Can you work these out from the model? Positions are in its coordinate system, mm. A direction names the side the tool comes from. Round coordinates to 2 decimals unless told otherwise and drop trailing zeros. Loops run counter-clockwise (first coordinate to the right, second up) from the corner with the lowest first, then second, coordinate; pieces in that order, holes last.
from build123d import *
from OCP.BRepFilletAPI import BRepFilletAPI_MakeChamfer

# Parameters (mm, degrees)
BOSS_EXTRUDE1_DEPTH             = 2
BOSS_EXTRUDE2_REACH             = 41.681
SKETCH2_W                       = 18.31765306
SKETCH2_H                       = 6
BOSS_EXTRUDE2_DIRECTION_2_DEPTH = 10
CUT_EXTRUDE1_DEPTH              = 8
CUT_EXTRUDE2_DEPTH              = 39.837136106
CUT_EXTRUDE2_DEPTH_BACK         = 39.837136106
SKETCH4_W                       = 8
SKETCH4_H                       = 2
CHAMFER1_SIZE                   = 2
CHAMFER2_SIZE                   = 10
CHAMFER2_SIZE2                  = 5.773502692
FILLET1_START                   = -2
FILLET1_DEPTH                   = 4
FILLET1_2_DEPTH                 = 4
BOSS_EXTRUDE3_START             = -6
SKETCH5_W                       = 10
SKETCH5_H                       = 1.6
BOSS_EXTRUDE3_DEPTH             = 10.5


with BuildPart() as part:
    # Sketch1 → Boss-Extrude1 (new, symmetric)
    with BuildSketch(Plane(origin=(0, 0, 0), x_dir=(1, 0, 0), z_dir=(0, 1, 0))):
        Polygon((-8, 0), (0, 0), (0, -1.2), (-9.15882653, -1.2), (-9.606841403, 11.62946737), (-13.196767517, 17.374550089), (-21.640774961, 32), (-20.255134315, 32), (-12.168010072, 17.992689924), (-8.41879396, 11.992689924), align=None)
    boss_extrude1 = extrude(amount=BOSS_EXTRUDE1_DEPTH, both=True)

    # Mirror1: Boss-Extrude1 across plane
    add(boss_extrude1.mirror(Plane(origin=(0, 2, 0), x_dir=(0, 0, 1), z_dir=(-1, 0, 0))))

    # Boss-Extrude2: up to this face of the body (flat: up to its plane)
    boss_extrude2_end = Plane(part.part.faces().sort_by_distance((0, 0, 0))[0])
    # Sketch2 → Boss-Extrude2 (add, up to the picked face)
    with BuildSketch(Plane.XY.offset(1.2), mode=Mode.PRIVATE) as boss_extrude2_sk1:
        with Locations((0, -1)):
            Rectangle(SKETCH2_W, SKETCH2_H)
    boss_extrude2_tool1 = split(extrude(boss_extrude2_sk1.sketch, amount=-BOSS_EXTRUDE2_REACH, mode=Mode.PRIVATE), bisect_by=boss_extrude2_end, keep=Keep.BOTH, mode=Mode.PRIVATE)
    add(boss_extrude2_tool1.solids().sort_by(Axis((0, -1, 1.2), (0, 0, -1)))[0])

    # Sketch2 → Boss-Extrude2 direction 2 (add)
    with BuildSketch(Plane.XY.offset(1.2)):
        with Locations((0, -1)):
            Rectangle(SKETCH2_W, SKETCH2_H)
    extrude(amount=BOSS_EXTRUDE2_DIRECTION_2_DEPTH)

    # Sketch3 → Cut-Extrude1 (cut)
    with BuildSketch(Plane.XY.offset(11.2)):
        with BuildLine():
            Line((-1.5, 1.826658805), (-1.5, 2))
            Line((-1.5, 2), (1.5, 2))
            Line((1.5, 2), (1.5, 1.826658805))
            ThreePointArc((1.5, 1.826658805), (3.2, -1), (1.5, -3.826658805))
            Line((1.5, -3.826658805), (1.5, -4))
            Line((1.5, -4), (-1.5, -4))
            Line((-1.5, -4), (-1.5, -3.826658805))
            ThreePointArc((-1.5, -3.826658805), (-3.2, -1), (-1.5, 1.826658805))
        make_face()
    extrude(amount=-CUT_EXTRUDE1_DEPTH, mode=Mode.SUBTRACT)

    # Sketch4 → Cut-Extrude2 (cut, two sides: drawn at the far end of the back side and taken through both)
    with BuildSketch(Plane(origin=(0, 0, 0), x_dir=(1, 0, 0), z_dir=(0, 1, 0)).offset(-CUT_EXTRUDE2_DEPTH_BACK)):
        with Locations((0, -4.2)):
            Rectangle(SKETCH4_W, SKETCH4_H)
    extrude(amount=CUT_EXTRUDE2_DEPTH + CUT_EXTRUDE2_DEPTH_BACK, mode=Mode.SUBTRACT)

    # Chamfer1
    chamfer1_edges = [part.edges().sort_by_distance(p)[0] for p in [
        (8.579413265, -2, 0),
        (-8.579413265, -2, 0),
    ]]
    chamfer(chamfer1_edges, length=CHAMFER1_SIZE - 0.0001)  # a hair under: the kernel refuses the full size

    # Chamfer2: one chamfer whose edges measure the first distance from different faces: ONE call of the kernel's chamfer builder (chamfer() names one face for all edges)
    chamfer2_edges_1 = [part.edges().sort_by_distance(p)[0] for p in [
        (9.15882653, -1, 11.2),
    ]]
    chamfer2_side_1 = [part.faces().sort_by_distance(p)[0] for p in [
        (9.15882653, -1.126288177, 5.77807488),
    ]]
    chamfer2_edges_2 = [part.edges().sort_by_distance(p)[0] for p in [
        (-9.15882653, -1, 11.2),
    ]]
    chamfer2_side_2 = [part.faces().sort_by_distance(p)[0] for p in [
        (-9.15882653, -1.126288177, 5.77807488),
    ]]
    chamfer2 = BRepFilletAPI_MakeChamfer(part.part.solid().wrapped)
    for e in chamfer2_edges_1:
        chamfer2.Add(CHAMFER2_SIZE, CHAMFER2_SIZE2, e.wrapped, chamfer2_side_1[0].wrapped)  # the first distance lies on this face
    for e in chamfer2_edges_2:
        chamfer2.Add(CHAMFER2_SIZE, CHAMFER2_SIZE2, e.wrapped, chamfer2_side_2[0].wrapped)  # the first distance lies on this face
    add(Compound.cast(chamfer2.Shape()), mode=Mode.REPLACE)

    # Fillet1: read off the stored shape, not the designer's step
    # Fillet1 outline → Fillet1 (cut)
    with BuildSketch(Plane(origin=(0, 0, 0), x_dir=(1, 0, 0), z_dir=(0, 1, 0)).offset(FILLET1_START)):
        with BuildLine():
            Line((13.196767517, 17.374550089), (13.327680504, 17.601298033))
            ThreePointArc((13.327680504, 17.601298033), (13.194808958, 17.37572691), (13.05802089, 17.15250907))
            Line((13.05802089, 17.15250907), (13.196767517, 17.374550089))
        make_face()
        with BuildLine():
            ThreePointArc((8.278524581, 7.975900449), (8.924815647, 11.837983569), (10.548665544, 15.401196962))
            Line((10.548665544, 15.401196962), (8.41879396, 11.992689924))
            Line((8.41879396, 11.992689924), (8.278524581, 7.975900449))
        make_face()
        with BuildLine():
            Line((-13.196767517, 17.374550089), (-13.05802089, 17.15250907))
            ThreePointArc((-13.05802089, 17.15250907), (-13.194808958, 17.37572691), (-13.327680504, 17.601298033))
            Line((-13.327680504, 17.601298033), (-13.196767517, 17.374550089))
        make_face()
        with BuildLine():
            Line((-8.41879396, 11.992689924), (-10.548665544, 15.401196962))
            ThreePointArc((-10.548665544, 15.401196962), (-8.924815647, 11.837983569), (-8.278524581, 7.975900449))
            Line((-8.278524581, 7.975900449), (-8.41879396, 11.992689924))
        make_face()
    extrude(amount=FILLET1_DEPTH, mode=Mode.SUBTRACT)

    # Fillet1 2 outline → Fillet1 2 (add)
    with BuildSketch(Plane(origin=(0, 0, 0), x_dir=(1, 0, 0), z_dir=(0, 1, 0)).offset(FILLET1_START)):
        with BuildLine():
            ThreePointArc((9.466572023, 7.612677895), (10.112863089, 11.474761015), (11.736712986, 15.037974408))
            Line((11.736712986, 15.037974408), (9.606841403, 11.62946737))
            Line((9.606841403, 11.62946737), (9.466572023, 7.612677895))
        make_face()
        with BuildLine():
            ThreePointArc((12.298923059, 18.219437869), (12.166051513, 17.993866745), (12.029263444, 17.770648906))
            Line((12.029263444, 17.770648906), (12.168010072, 17.992689924))
            Line((12.168010072, 17.992689924), (12.298923059, 18.219437869))
        make_face()
        with BuildLine():
            Line((-9.606841403, 11.62946737), (-11.736712986, 15.037974408))
            ThreePointArc((-11.736712986, 15.037974408), (-10.112863089, 11.474761015), (-9.466572023, 7.612677895))
            Line((-9.466572023, 7.612677895), (-9.606841403, 11.62946737))
        make_face()
        with BuildLine():
            ThreePointArc((-12.029263444, 17.770648906), (-12.166051513, 17.993866745), (-12.298923059, 18.219437869))
            Line((-12.298923059, 18.219437869), (-12.168010072, 17.992689924))
            Line((-12.168010072, 17.992689924), (-12.029263444, 17.770648906))
        make_face()
    extrude(amount=FILLET1_2_DEPTH)

    # Sketch5 → Boss-Extrude3 (add)
    with BuildSketch(Plane.XZ.offset(4).offset(BOSS_EXTRUDE3_START)):
        with Locations((0, 0.8)):
            Rectangle(SKETCH5_W, SKETCH5_H)
    extrude(amount=BOSS_EXTRUDE3_DEPTH)


solid = part.part
(1) If we section it at D-D, the plane z = -22: List the corners of the cut face in (x, y) for me, then the cut area to 3 significant figures.
Worked answers:
outline: (-15.87, -2) - (-14.48, -2) - (-14.48, 2) - (-15.87, 2) - close; (14.48, -2) - (15.87, -2) - (15.87, 2) - (14.48, 2) - close
area: 11.1 mm2
(2) If we mould it in two halves opening along Z, with no side actions, what happens to faces 1 (the flat face through (-3.6, -1, 5.2)), 2 (the flat face through (0, -4, 3)), 3 (the flat face through (17.426, 0.028, -24.7))? For each: released by +Z, released by -Z, zero draft, split by the parting line, or undercut.
Worked answers:
face 1: undercut
face 2: zero draft
face 3: released by +Z
(3) Will these pins go through, and if not, where does the flat tip stop? P1, Ø2, axis at y = -1, z = 4, coming from the -X side; P2, Ø3, axis at y = -7, z = -1, coming from the -X side; P3, Ø2, axis at y = -3.5, z = 0.5, coming from the -X side.
Worked answers:
P1: stops at x = -8.12
P2: stops at x = -5
P3: stops at x = -9.16
(4) If we section it at B-B, the plane z = 4: List the corners of the cut face in (x, y) for me.
Worked answers:
outline: (-7.54, -4) - (-4, -4) - (-4, 2) - (-7.54, 2) - close; (4, -4) - (7.54, -4) - (7.54, 2) - (4, 2) - close
(5) If I drill on line 1 (Y direction, x = 10, z = -13); line 2 (Z direction, x = -2.5, y = -0.25); line 3 (X direction, y = -8, z = 1), over which ranges is the centre line in solid material (lowest first)?
Worked answers:
line 1: y = -2 to 2
line 2: z = 0 to 3.2
line 3: x = -5 to 5
(6) For faces 4 (the flat face through (9.159, -3, 0)), 5 (the flat face through (4, -1, 4)), 6 (the flat face through (6.23, -1.04, 6.27)), 7 (the cylindrical face through (3.2, -1, 8.2)), 8 (the flat face through (11.3, 0, -16.6)), which set-ups out of +Z, -Z, +X, -X, +Y, -Y let a thin tool reach every point of the face, with its end or its side?
Worked answers:
face 4: +Z, -Z, +X, -Y
face 5: +Y, -Y
face 6: +Z, +X, +Y, -Y
face 7: +Z
face 8: -Z, +Y, -Y
(7) If we section it at A-A, the plane x = -2.5: List the corners of the cut face in (y, z) for me, then the cut area to 3 significant figures.
Worked answers:
outline: (-8.5, 0) - (2, 0) - (2, 3.2) - (-4, 3.2) - (-4, 1.6) - (-8.5, 1.6) - close; (-4, 5.2) - (-3, 5.2) - (-3, 11.2) - (-4, 11.2) - close; (1, 5.2) - (2, 5.2) - (2, 11.2) - (1, 11.2) - close
area: 38.4 mm2
